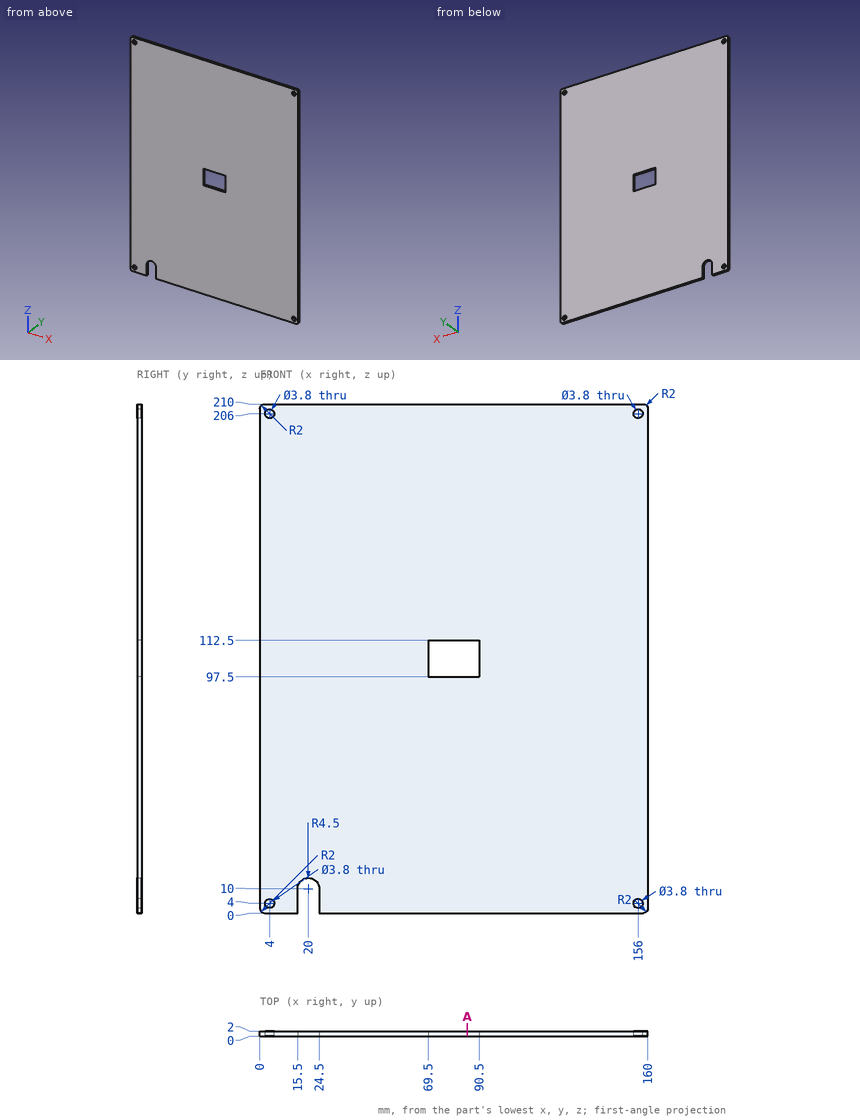
Can you work these out from the drawing? Everything is in mm from the part's minimum corner. Coordinates: 2 decimals unless noted, no trailing zeros. Loops run counter-clockwise (first coordinate to the right, second up) from the corner with the lowest first, then second, coordinate; pieces in that order, holes last. Notation, with made-up numbers: (89.25, 62) - (103.25, 62) arc R14 cw to (103.25, 73) - close; hole circle Ø1 at (-36.75, -10). An arc over 180 degrees is marked (long way). Put each result on its own line as item: value. Start each with the question number.
Item 1: Suppose I cut it at A-A (x = 85.5). Please give me the cut outline in (y, z), and give its area (3 significant figures).
Item 2: If I drill on line 1 along Z through (x, y) = (156, 1.1); line 2 along X through (y, z) = (1.5, 206); line 3 along X through (y, z) = (1.9, 111.5), over which ranges is the centre line in solid material (lowest first)?
Item 3: For pin 1 (2.5 mm diameter, centred on x = 4, z = 4, fed in from +Y), with a flat end and sliding along its axis, tell me the tip position at first contact or that it passes through.
Here are the results:
1. outline: (0, 0) - (2, 0) - (2, 97.5) - (0, 97.5) - close; (0, 112.5) - (2, 112.5) - (2, 210) - (0, 210) - close
1. area: 390 mm²
2. line 1: 0 to 2.1, 5.9 to 204.1, 207.9 to 210
2. line 2: 0 to 2.1, 5.9 to 154.1, 157.9 to 160
2. line 3: 0 to 69.5, 90.5 to 160
3. pin 1: through
